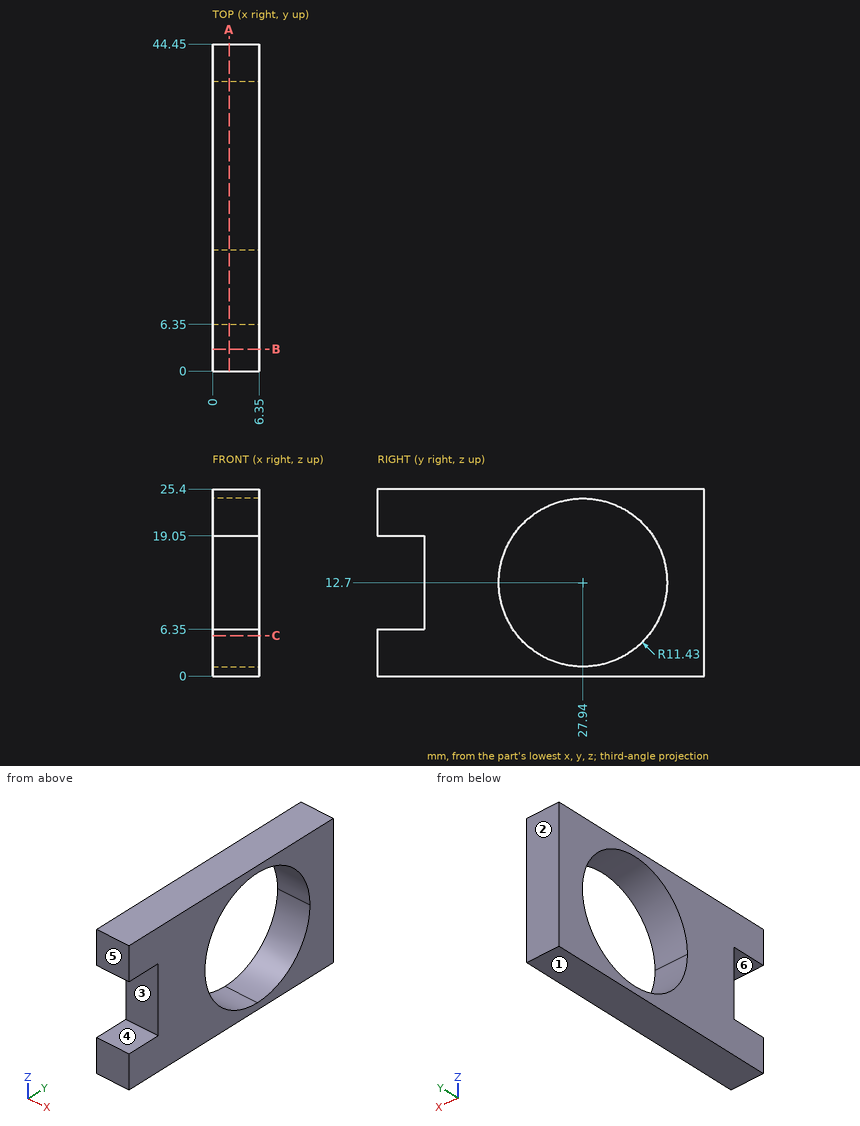
Here's the drawing with two shaded views (mm, measured from the low corner). I have some questions. A direction names the side the tool comes from. Round coordinates to 2 decimals unless told otherwise and drop trailing zeros. Loops run counter-clockwise (first coordinate to the right, second up) from the corner with the lowest first, then second, coordinate; pieces in that order, holes last.
1. For the marked faces 5 and 6, which set-ups out of +Z, -Z, +X, -X, +Y, -Y let a thin tool reach every point of the face, with its end or its side?
Answers:
face 5: +Z, -Z, +X, -X, -Y
face 6: +X, -X, -Y
2. If I drill on probe 1 along Y at (x, z) = (1.25, 12.25); probe 2 along Y at (x, z) = (1, 11); probe 3 along Z at (x, y) = (1.75, 32.5), over which ranges is the centre line in solid material (lowest first)?
Answers:
probe 1: y = 6.35 to 16.52, 39.36 to 44.45
probe 2: y = 6.35 to 16.64, 39.24 to 44.45
probe 3: z = 0 to 2.22, 23.18 to 25.4
3. Suppose I cut it at A-A, the plane x = 2.25. Please give me the cut outline in (y, z).
Answers:
outline: (0, 0) - (44.45, 0) - (44.45, 25.4) - (0, 25.4) - (0, 19.05) - (6.35, 19.05) - (6.35, 6.35) - (0, 6.35) - close; hole circle Ø22.86 at (27.94, 12.7)
4. Will this pin go through, and if not, where does the flat tip stop? pin 1 (1.9 mm diameter, centred on x = 4.5, z = 12, fed in from -Y).
Answers:
pin 1: stops at y = 6.35
5. Suppose I cut it at C-C, the plane z = 5.5. Please give me the cut outline in (x, y), and give its area (3 significant figures).
Answers:
outline: (0, 0) - (6.35, 0) - (6.35, 19.06) - (0, 19.06) - close; (0, 36.82) - (6.35, 36.82) - (6.35, 44.45) - (0, 44.45) - close
area: 170 mm2
6. Suppose I cut it at B-B, the plane y = 3. Please give me the cut outline in (x, z).
Answers:
outline: (0, 0) - (6.35, 0) - (6.35, 6.35) - (0, 6.35) - close; (0, 19.05) - (6.35, 19.05) - (6.35, 25.4) - (0, 25.4) - close
7. Thinking about a two-plate mould opening in Z: for the marked faces 1, 2, 3 and 4, which applies, released by +Z, released by -Z, zero draft, split by the parting line, or undercut?
Answers:
face 1: released by -Z
face 2: zero draft
face 3: undercut
face 4: undercut
